from build123d import *

# Parameters (mm, degrees)
SKETCH1_W          = 30.48
SKETCH1_H          = 12.7
CUT_EXTRUDE1_DEPTH = 8.382
CUT_EXTRUDE2_DEPTH = 5.318
CUT_EXTRUDE3_DEPTH = 8.382
CUT_EXTRUDE4_DEPTH = 5.318
CUT_EXTRUDE5_DEPTH = 8.382
CUT_EXTRUDE6_DEPTH = 5.318
CUT_EXTRUDE7_DEPTH = 8.382
CUT_EXTRUDE8_DEPTH = 5.318
HOLE1_D            = 6.35
HOLE1_DEPTH        = 12.7
HOLE1_CBORE_D      = 50.8
HOLE1_CBORE_DEPTH  = 0.381
CHAMFER1_SIZE      = 0.254


with BuildPart() as part:
    # Sketch1 → Revolve1 (revolve)
    with BuildSketch(Plane(origin=(0, 0, 0), x_dir=(-1, 0, 0), z_dir=(0, 0, -1))):
        with Locations((-15.24, 0)):
            Rectangle(SKETCH1_W, SKETCH1_H)
    revolve(axis=Axis((0, -6.35, 0), (0, 1, 0)))

    # Sketch2 → Cut-Extrude1 (cut)
    with BuildSketch(Plane(origin=(0, 6.35, 0), x_dir=(-1, 0, 0), z_dir=(0, 1, 0))):
        with BuildLine():
            Line((5.1562, -30.040705743), (5.1562, -11.938))
            ThreePointArc((5.1562, -11.938), (0, -6.7818), (-5.1562, -11.938))
            Line((-5.1562, -11.938), (-5.1562, -30.040705743))
            ThreePointArc((-5.1562, -30.040705743), (0, -30.48), (5.1562, -30.040705743))
        make_face()
    extrude(amount=-CUT_EXTRUDE1_DEPTH, mode=Mode.SUBTRACT)

    # Sketch3 → Cut-Extrude2 (cut, through all)
    with BuildSketch(Plane(origin=(0, -2.032, 0), x_dir=(-1, 0, 0), z_dir=(0, 1, 0))):
        with BuildLine():
            Line((3.3655, -30.293626553), (3.3655, -11.938))
            ThreePointArc((3.3655, -11.938), (0, -8.5725), (-3.3655, -11.938))
            Line((-3.3655, -11.938), (-3.3655, -30.293626553))
            ThreePointArc((-3.3655, -30.293626553), (0, -30.48), (3.3655, -30.293626553))
        make_face()
    extrude(amount=-CUT_EXTRUDE2_DEPTH, mode=Mode.SUBTRACT)

    # Sketch4 → Cut-Extrude3 (cut)
    with BuildSketch(Plane(origin=(0, 6.35, 0), x_dir=(-1, 0, 0), z_dir=(0, 1, 0))):
        with BuildLine():
            Line((-30.040705743, -5.1562), (-11.938, -5.1562))
            ThreePointArc((-11.938, -5.1562), (-6.7818, 0), (-11.938, 5.1562))
            Line((-11.938, 5.1562), (-30.040705743, 5.1562))
            ThreePointArc((-30.040705743, 5.1562), (-30.48, 0), (-30.040705743, -5.1562))
        make_face()
    extrude(amount=-CUT_EXTRUDE3_DEPTH, mode=Mode.SUBTRACT)

    # Sketch5 → Cut-Extrude4 (cut, through all)
    with BuildSketch(Plane(origin=(0, -2.032, 0), x_dir=(-1, 0, 0), z_dir=(0, 1, 0))):
        with BuildLine():
            Line((-30.293626553, -3.3655), (-11.938, -3.3655))
            ThreePointArc((-11.938, -3.3655), (-8.5725, 0), (-11.938, 3.3655))
            Line((-11.938, 3.3655), (-30.293626553, 3.3655))
            ThreePointArc((-30.293626553, 3.3655), (-30.48, 0), (-30.293626553, -3.3655))
        make_face()
    extrude(amount=-CUT_EXTRUDE4_DEPTH, mode=Mode.SUBTRACT)

    # Sketch6 → Cut-Extrude5 (cut)
    with BuildSketch(Plane(origin=(0, 6.35, 0), x_dir=(-1, 0, 0), z_dir=(0, 1, 0))):
        with BuildLine():
            Line((-5.1562, 30.040705743), (-5.1562, 11.938))
            ThreePointArc((-5.1562, 11.938), (0, 6.7818), (5.1562, 11.938))
            Line((5.1562, 11.938), (5.1562, 30.040705743))
            ThreePointArc((5.1562, 30.040705743), (0, 30.48), (-5.1562, 30.040705743))
        make_face()
    extrude(amount=-CUT_EXTRUDE5_DEPTH, mode=Mode.SUBTRACT)

    # Sketch7 → Cut-Extrude6 (cut, through all)
    with BuildSketch(Plane(origin=(0, -2.032, 0), x_dir=(-1, 0, 0), z_dir=(0, 1, 0))):
        with BuildLine():
            Line((-3.3655, 30.293626553), (-3.3655, 11.938))
            ThreePointArc((-3.3655, 11.938), (0, 8.5725), (3.3655, 11.938))
            Line((3.3655, 11.938), (3.3655, 30.293626553))
            ThreePointArc((3.3655, 30.293626553), (0, 30.48), (-3.3655, 30.293626553))
        make_face()
    extrude(amount=-CUT_EXTRUDE6_DEPTH, mode=Mode.SUBTRACT)

    # Sketch8 → Cut-Extrude7 (cut)
    with BuildSketch(Plane(origin=(0, 6.35, 0), x_dir=(-1, 0, 0), z_dir=(0, 1, 0))):
        with BuildLine():
            Line((30.040705743, 5.1562), (11.938, 5.1562))
            ThreePointArc((11.938, 5.1562), (6.7818, 0), (11.938, -5.1562))
            Line((11.938, -5.1562), (30.040705743, -5.1562))
            ThreePointArc((30.040705743, -5.1562), (30.48, 0), (30.040705743, 5.1562))
        make_face()
    extrude(amount=-CUT_EXTRUDE7_DEPTH, mode=Mode.SUBTRACT)

    # Sketch9 → Cut-Extrude8 (cut, through all)
    with BuildSketch(Plane(origin=(0, -2.032, 0), x_dir=(-1, 0, 0), z_dir=(0, 1, 0))):
        with BuildLine():
            Line((30.293626553, 3.3655), (11.938, 3.3655))
            ThreePointArc((11.938, 3.3655), (8.5725, 0), (11.938, -3.3655))
            Line((11.938, -3.3655), (30.293626553, -3.3655))
            ThreePointArc((30.293626553, -3.3655), (30.48, 0), (30.293626553, 3.3655))
        make_face()
    extrude(amount=-CUT_EXTRUDE8_DEPTH, mode=Mode.SUBTRACT)

    # Hole1
    with Locations(Plane(origin=(0, -6.35, 0), x_dir=(-1, 0, 0), z_dir=(0, -1, 0))):
        with Locations((0, 0)):
            CounterBoreHole(HOLE1_D / 2, HOLE1_CBORE_D / 2, HOLE1_CBORE_DEPTH, depth=HOLE1_DEPTH)

    # Chamfer1
    chamfer1_edges = [part.edges().sort_by_distance(p)[0] for p in [
        (-3.175, -5.969, 0),
        (-3.175, 6.35, 0),
    ]]
    chamfer(chamfer1_edges, length=CHAMFER1_SIZE)


solid = part.part
CAD build for the part. Positions are in the model's coordinates, mm. A direction names the side the tool comes from. Round coordinates to 2 decimals unless told otherwise and drop trailing zeros. Order: outer loops, then holes, each group sorted by start corner. A loop starts at its lowest first (then second) coordinate and runs counter-clockwise, first axis right, second up. Notation, with made-up numbers: M 83.5,-16.5 L 122.5,-16.5 A13 ccw 122.5,-11.5 Z; hole C 70.5,48.5 d7. An arc over 180 degrees is marked long. Use one line per item in the form item = value.
Q1. Probe L1, parallel to Z at x = 0, y = 0.75 (3 decimals); L2, parallel to Y at x = -16.5, z = -13.5. List the from-to ranges inside material, lowest first.
Recorded:
L1 = -6.782 to -3.175, 3.175 to 6.782
L2 = -5.97 to 6.35
Q2. Saw through at C-C on y = 0.75. Give the cut face in (x, z) (3 decimals), then the cut area to 3 significant figures.
Recorded:
outline = M -30.041,-5.156 A30.48 ccw -5.156,-30.041 L -5.156,-11.938 A5.156 cw 5.156,-11.938 L 5.156,-30.041 A30.48 ccw 30.041,-5.156 L 11.938,-5.156 A5.156 cw 11.938,5.156 L 30.041,5.156 A30.48 ccw 5.156,30.041 L 5.156,11.938 A5.156 cw -5.156,11.938 L -5.156,30.041 A30.48 ccw -30.041,5.156 L -11.938,5.156 A5.156 cw -11.938,-5.156 Z; hole C 0,0 d6.35
area = 1,960 mm^2
Q3. Saw through at D-D on z = -7.5. Give the cut face in (x, y), then the cut area to 3 significant figures.
Recorded:
outline = M -29.54,-6.35 L -24.27,-6.35 L -24.27,-5.97 L 24.27,-5.97 L 24.27,-6.35 L 29.54,-6.35 L 29.54,6.35 L 2.62,6.35 L 2.62,-2.03 L -2.62,-2.03 L -2.62,6.35 L -29.54,6.35 Z
area = 688 mm^2
Q4. Which spindle directions (+Z, -Z, +X, -X, +Y, -Y) get a long thin tool onto all of the face, cutting with end or side? Do faces 1 (the flat face through (-21, -4, 3.366)), 2 (the cylindrical face through (-0.113, 2.218, -6.783)), 3 (the flat face through (21, 2, 5.156)), 4 (the cylindrical face through (-17.8, -6.16, 18.12)). Say none if no direction does.
Recorded:
face_1 = -X, +Y, -Y
face_2 = -Z, +Y
face_3 = +X, +Y
face_4 = -Y
Q5. Two-plate mould, pull along Z, no slides. Class faces 5 (the flat face through (4, -2.032, -18)), 6 (the cylindrical face through (0.074, -3.973, 8.573)), 7 (the flat face through (-21, -4, -3.366)): +Z half, -Z half, draft (parallel to the pull), parting line (faces both ways), or undercut.
Recorded:
face_5 = draft
face_6 = +Z half
face_7 = undercut
Q6. Flat gauge pins, fed straight in: P1, Ø3, axis at x = 17, z = -2, coming from the +Y side; P2, Ø10, axis at x = -6.5, z = 15.5, coming from the -Y side; P3, Ø1, axis at x = 8.5, y = -5, coming from the +Z side. Where does each tip first touch, or does it go through?
Recorded:
P1 = -2.03
P2 = -5.97
P3 = 29.41
